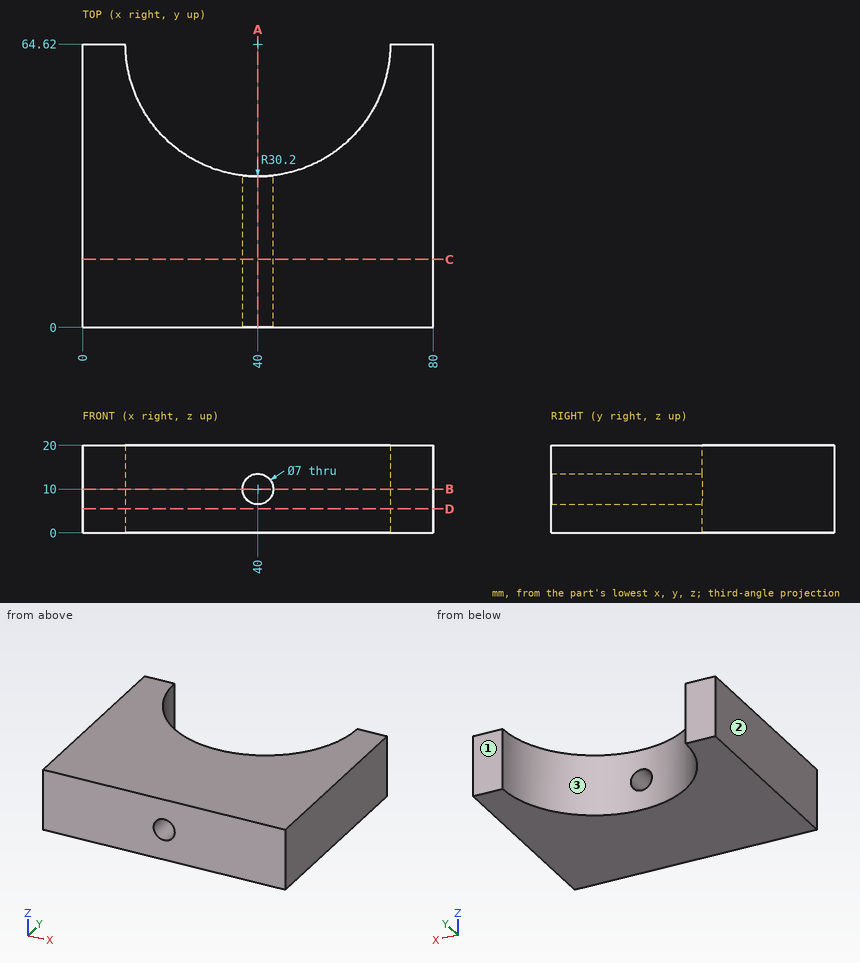
Can you work these out from the drawing? Everything is in mm from the part's minimum corner. Coordinates: 2 decimals unless noted, no trailing zeros. Loops run counter-clockwise (first coordinate to the right, second up) from the corner with the lowest first, then second, coordinate; pieces in that order, holes last.
1. Imagine slicing it at D-D, the plane z = 5.5. Please give me the cut outline in (x, y), and give its area (3 significant figures).
2. Imagine slicing it at A-A, the plane x = 40. Please give me the cut outline in (y, z).
3. I need wall thicknesses on L1, parallel to Z at x = 40, y = 16; L2, parallel to X at y = 30, z = 12.75; L3, parallel to Y at x = 32, z = 6.5. Which ranges of each line are inside material? Lowest first, please.
4. Imagine slicing it at C-C, the plane y = 15.5. Please give me the cut outline in (x, z).
5. For P1, Ø8, axis at x = 40, z = 10, coming from the +Y side; P2, Ø2, axis at x = 39, z = 12, coming from the +Y side, each with a flat end and sliding along its axis, tell me the tip position at first contact or that it passes through.
6. If we mould it in two halves opening along X, with no side actions, what happens to the marked faces 1, 2 and 3? For each: pulls with the +X half, pulls with the -X half, needs draft (parallel to the pull), parting line crosses it, or undercut.
7. Imagine slicing it at B-B, the plane z = 10. Please give me the cut outline in (x, y).
Taken from the geometry:
1. outline: (0, 0) - (80, 0) - (80, 64.62) - (70.2, 64.62) arc R30.2 cw to (9.8, 64.62) - (0, 64.62) - close
1. area: 3,740 mm2
2. outline: (0, 0) - (34.42, 0) - (34.42, 6.5) - (0, 6.5) - close; (0, 13.5) - (34.42, 13.5) - (34.42, 20) - (0, 20) - close
3. L1: z = 0 to 6.5, 13.5 to 20
3. L2: x = 0 to 37.83, 42.17 to 80
3. L3: y = 0 to 35.5
4. outline: (0, 0) - (80, 0) - (80, 20) - (0, 20) - close; hole circle Ø7 at (40, 10)
5. P1: stops at y = 34.69
5. P2: passes through
6. face 1: needs draft
6. face 2: pulls with the -X half
6. face 3: undercut
7. outline: (0, 0) - (36.5, 0) - (36.5, 34.62) arc R30.2 cw to (9.8, 64.62) - (0, 64.62) - close; (43.5, 0) - (80, 0) - (80, 64.62) - (70.2, 64.62) arc R30.2 cw to (43.5, 34.62) - close
